Part model, mm, in its own coordinate system. A direction names the side the tool comes from. Round coordinates to 2 decimals unless told otherwise and drop trailing zeros. Loops run counter-clockwise (first coordinate to the right, second up) from the corner with the lowest first, then second, coordinate; pieces in that order, holes last.
(1) Cut at B-B on x = -57.5. List the corners of the cut face in (y, z), then the cut area to 3 significant figures.
(2) Tool access for faces 4 (the face through (32.5, 0, 5)), 5 (the face through (55, -39, 7)), 6 (the face through (-52.5, 37, 9)), 7 (the face through (-55, 39, 7)), 8 (the face through (52.5, -37, 9)): list every direction of +Z, -Z, +X, -X, +Y, -Y with a clear straight run to the whole face (end or side of a thin tool).
(3) Mould opens along Y. For faces 1 (the face through (13, 24, 0)), 2 (the face through (-59.81, -39.04, 8.52)), 3 (the face through (57.6, 45, 8.5)) say: +Y half, -Y half, draft (parallel to the pull), parting line (faces both ways), or undercut.
(4) Cut at D-D on z = 5. List the corners of the cut face in (x, y).
(5) Cut at C-C on x = -8.5. List the corners of the cut face in (y, z), then the cut area to 3 significant figures.
(6) Flat gauge pins, fed straight in: pin 1 (5 mm diameter, centred on x = -10.5, z = 5, fed in from -Y); pin 2 (8 mm diameter, centred on x = -57.5, y = -40, fed in from -Z); pin 3 (5 mm diameter, centred on y = 2.5, z = 3, fed in from -X). Where does each tip first touch, or does it go through?
(7) Cut at A-A on x = 57.5. List the corners of the cut face in (y, z).
(8) Probe probe 1 along Y at (x, z) = (57.5, 7.7); probe 2 along X at (y, z) = (40, 8.25); probe 3 along Y at (x, z) = (-57.5, 7.6). List the from-to ranges inside material, lowest first.
Autodesk Fusion 360 part; units mm, degrees
sketch "Sketch1" plane through (0, 0, 0) normal (0, 0, 1) x (1, 0, 0)
  line L0 (62.5, -35) -> (-62.5, -35)
  line L1 (-62.5, -35) -> (-62.5, 35)
  line L2 (-62.5, 35) -> (62.5, 35)
  line L3 (62.5, 35) -> (62.5, -35)
  line L4 (62.5, -35) -> (-62.5, 35) construction
  line L5 (-62.5, -35) -> (62.5, 35) construction
  dimension "d1" = 125
  dimension "d2" = 70
extrude "Extrude1" add sketch "Sketch1" along normal blind 10
sketch "Sketch2" plane through (0, 0, 10) normal (0, 0, 1) x (-1, 0, 0)
  line L0 (-62.5, -35) -> (62.5, -35)
  line L1 (62.5, -35) -> (62.5, 35)
  line L2 (62.5, 35) -> (-62.5, 35)
  line L3 (-62.5, 35) -> (-62.5, -35)
sketch "Sketch3" plane through (0, 0, 0) normal (0, 0, -1) x (1, 0, 0)
  line L0 (-62.5, -35) -> (62.5, -35)
  line L1 (62.5, -35) -> (62.5, 35)
  line L2 (62.5, 35) -> (-62.5, 35)
  line L3 (-62.5, 35) -> (-62.5, -35)
  line L4 (-62.5, 0) -> (-62.5, 17.5)
  line L5 (-62.5, 0) -> (-62.5, -17.5)
  line L6 (-62.5, 17.5) -> (32.5, 17.5)
  line L7 (32.5, 17.5) -> (32.5, -17.5)
  line L8 (-62.5, -17.5) -> (32.5, -17.5)
  dimension "d5" = 17.5
  dimension "d6" = 17.5
  dimension "d7" = 95
  dimension "d8" = 35
extrude "Extrude2" cut sketch "Sketch3" against normal blind 8 contours L3 L4 L5 L6 L7 L8
extrude "Extrude3" cut 1 faces at (-30.8333, -5.8333, 8) along direction (0, 0, 1) blind 30
sketch "Sketch4" plane through (0, 0, 10) normal (0, 0, 1) x (-1, 0, 0)
  line L0 (62.5, -35) -> (52.5, -35)
  line L1 (52.5, -35) -> (52.5, -40)
  line L2 (62.5, -40) -> (62.5, -35)
  arc A0 (57.5, -45) -> (62.5, -40) centre (57.5, -40) ccw
  arc A1 (52.5, -40) -> (57.5, -45) centre (57.5, -40) ccw
  circle A2 centre (57.5, -40) radius 2.5
  point P0 (62.5, -45)
  dimension "d13" = 10
  dimension "d14" = 10
  dimension "d15" = 5
  dimension "d16" = 5
  dimension "d17" = 5
extrude "Extrude4" add sketch "Sketch4" against normal blind 3
mirror "Mirror1" about plane through (0, 0, 0) normal (1, 0, 0) of "Extrude4"
mirror "Mirror2" about plane through (0, 0, 0) normal (0, 1, 0) of "Extrude4", "Mirror1"
equation "d5 = ( 35 / 2 ) * 1 mm"
Final values:
1. outline: (-45, 7) - (-42.5, 7) - (-42.5, 10) - (-45, 10) - close; (-37.5, 7) - (-35, 7) - (-35, 0) - (-17.5, 0) - (-17.5, 10) - (-37.5, 10) - close; (17.5, 0) - (35, 0) - (35, 7) - (37.5, 7) - (37.5, 10) - (17.5, 10) - close; (42.5, 7) - (45, 7) - (45, 10) - (42.5, 10) - close
1. area: 380 mm2
2. face 4: +Z, -Z, -X
2. face 5: -Z, +X, -X, -Y
2. face 6: +Z, -Z, +Y
2. face 7: -Z, +X, -X, +Y
2. face 8: +Z, -Z, -Y
3. face 1: draft
3. face 2: undercut
3. face 3: +Y half
4. outline: (-62.5, -35) - (62.5, -35) - (62.5, 35) - (-62.5, 35) - (-62.5, 17.5) - (32.5, 17.5) - (32.5, -17.5) - (-62.5, -17.5) - close
5. outline: (-35, 0) - (-17.5, 0) - (-17.5, 10) - (-35, 10) - close; (17.5, 0) - (35, 0) - (35, 10) - (17.5, 10) - close
5. area: 350 mm2
6. pin 1: stops at y = -35
6. pin 2: stops at z = 7
6. pin 3: stops at x = 32.5
7. outline: (-45, 7) - (-42.5, 7) - (-42.5, 10) - (-45, 10) - close; (-37.5, 7) - (-35, 7) - (-35, 0) - (35, 0) - (35, 7) - (37.5, 7) - (37.5, 10) - (-37.5, 10) - close; (42.5, 7) - (45, 7) - (45, 10) - (42.5, 10) - close
8. probe 1: y = -45 to -42.5, -37.5 to 37.5, 42.5 to 45
8. probe 2: x = -62.5 to -60, -55 to -52.5, 52.5 to 55, 60 to 62.5
8. probe 3: y = -45 to -42.5, -37.5 to -17.5, 17.5 to 37.5, 42.5 to 45
